```python
from build123d import *

# Parameters (mm, degrees)
F0_R      = 7.25
F1_DEPTH  = 14
F3_R      = 3
F4_DEPTH  = 14.001
F6_R      = 12.75
F7_DEPTH  = 25
F8_R      = 3.95
F9_DEPTH  = 39.001
F10_R     = 12.75
F10_R_2   = 11.5
F11_DEPTH = 20
F13_DEPTH = 5
F14_R     = 3.95
F15_DEPTH = 6.5


with BuildPart() as f1:
    # F0 (on Front) → F1 (new body)
    with BuildSketch(Plane.XZ):
        Circle(F0_R)
    extrude(amount=F1_DEPTH)

    # F3 (on face) → F4 (cut, through all)
    with BuildSketch(Plane.XZ.offset(14)):
        Circle(F3_R)
    extrude(amount=-F4_DEPTH, mode=Mode.SUBTRACT)

    # F6 (on offset) → F7 (join)
    with BuildSketch(Plane(origin=(0, 0, 0), x_dir=(-1, 0, 0), z_dir=(0, 1, 0))):
        Circle(F6_R)
    extrude(amount=F7_DEPTH)

    # F8 (on face) → F9 (cut, through all)
    with BuildSketch(Plane(origin=(0, 25, 0), x_dir=(-1, 0, 0), z_dir=(0, 1, 0))):
        Circle(F8_R)
    extrude(amount=-F9_DEPTH, mode=Mode.SUBTRACT)

    # F10 (on face) → F11 (cut)
    with BuildSketch(Plane(origin=(0, 25, 0), x_dir=(-1, 0, 0), z_dir=(0, 1, 0))):
        Circle(F10_R)
        Circle(F10_R_2, mode=Mode.SUBTRACT)
    extrude(amount=-F11_DEPTH, mode=Mode.SUBTRACT)

    # F12 (on face) → F13 (join)
    with BuildSketch(Plane(origin=(0, 5, 0), x_dir=(-1, 0, 0), z_dir=(0, 1, 0))):
        with BuildLine():
            ThreePointArc((2, 12.5921602595), (0, 12.75), (-2, 12.5921602595))
            Line((-2, 12.5921602595), (-2, 11.3247516529))
            ThreePointArc((-2, 11.3247516529), (0, 11.5), (2, 11.3247516529))
            Line((2, 11.3247516529), (2, 12.5921602595))
        make_face()
        with BuildLine():
            Line((-2, -11.3247516529), (-2, -12.5921602595))
            ThreePointArc((-2, -12.5921602595), (0, -12.75), (2, -12.5921602595))
            Line((2, -12.5921602595), (2, -11.3247516529))
            ThreePointArc((2, -11.3247516529), (0, -11.5), (-2, -11.3247516529))
        make_face()
    extrude(amount=F13_DEPTH)

    # F14 (on face) → F15 (cut)
    with BuildSketch(Plane(origin=(0, 25, 0), x_dir=(-1, 0, 0), z_dir=(0, 1, 0))):
        Polygon((5.6975970229, 5.0613622835), (-1.5344698039, 7.4649449041), (-7.2320668267, 2.4035826206), (-5.6975970229, -5.0613622835), (1.5344698039, -7.4649449041), (7.2320668267, -2.4035826206), align=None)
        Circle(F14_R, mode=Mode.SUBTRACT)
    extrude(amount=-F15_DEPTH, mode=Mode.SUBTRACT)


solid = f1.part
```
CAD build for the part. Positions are in the model's coordinates, mm. A direction names the side the tool comes from. Round coordinates to 2 decimals unless told otherwise and drop trailing zeros. Order: outer loops, then holes, each group sorted by start corner. A loop starts at its lowest first (then second) coordinate and runs counter-clockwise, first axis right, second up. Notation, with made-up numbers: (29, 45.5) - (82, 45.5) arc R30 ccw to (82, 75.5) - close; hole circle Ø5 at (40, 12). An arc over 180 degrees is marked (long way). Answer in a Markdown table with one row per item. Add a question column.
(1) 3-axis set-ups, long thin cutter, end or side, ignore diameter. For faces 1 (the face through (3.35, -6.9, -6.43)), 2 (the face through (-2, 7, -12)), 3 (the face through (2, 7, 12)), 4 (the face through (2, 7, -12)), 5 (the face through (6.476, 21.796, -1.277)): which of +Z, -Z, +X, -X, +Y, -Y reach the whole face in a straight line?
(2) Probe L1, parallel to Z at x = 0, y = -5.5; L2, parallel to Y at x = -1.25, z = -5; L3, parallel to Y at x = 10, z = -1. List the from-to ranges inside material, lowest first. Write a range as [from, to].
(3) Band-saw the part on B-B on y = 4.5. List the corners of the cut face in (x, z).
(4) Band-saw the part on C-C on z = 0. List the corners of the cut face in (x, y), and give its area (3 significant figures).
(5) Mould opens along Z. For faces 6 (the face through (-12, 5, 0)), 7 (the face through (3.135, 2.477, -2.404)), 8 (the face through (2.493, 15.14, -11.227)) say: +Z half, -Z half, draft (parallel to the pull), parting line (faces both ways), or undercut.
(6) Band-saw the part on D-D on x = -10.5. List the corners of the cut face in (y, z), and give its area (3 significant figures).
(7) Drop flat-ended pins along their axis: pin 1 Ø12 at (x, y) = (-10, -7.5) entering from +Z; pin 2 Ø1 at (y, z) = (8, 12) entering from +X; pin 3 Ø8 at (y, z) = (3.5, -4.5) entering from +X. Give the stop position or say it passes through.
(8) Band-saw the part on A-A on x = 0. List the corners of the cut face in (y, z), and give its area (3 significant figures).
Data:
| question | item | result |
|---|---|---|
| 1 | face 1 | -Y |
| 1 | face 2 | -Z, -X, +Y |
| 1 | face 3 | +Z, +X, +Y |
| 1 | face 4 | -Z, +X, +Y |
| 1 | face 5 | +Y |
| 2 | L1 | z = [-7.25, -3.95], [3.95, 7.25] |
| 2 | L2 | y = [-14, 18.5] |
| 2 | L3 | y = [0, 25] |
| 3 | outline | circle Ø25.5 at (0, 0); hole circle Ø7.9 at (0, 0) |
| 4 | outline | (-12.75, 0) - (-7.25, 0) - (-7.25, -14) - (-3.95, -14) - (-3.95, 18.5) - (-6.74, 18.5) - (-6.74, 25) - (-11.5, 25) - (-11.5, 5) - (-12.75, 5) - close; (3.95, -14) - (7.25, -14) - (7.25, 0) - (12.75, 0) - (12.75, 5) - (11.5, 5) - (11.5, 25) - (6.74, 25) - (6.74, 18.5) - (3.95, 18.5) - close |
| 4 | area | 446 mm^2 |
| 5 | face 6 | draft |
| 5 | face 7 | undercut |
| 5 | face 8 | parting line |
| 6 | outline | (0, -7.23) - (5, -7.23) - (5, -4.69) - (25, -4.69) - (25, 4.69) - (5, 4.69) - (5, 7.23) - (0, 7.23) - close |
| 6 | area | 260 mm^2 |
| 7 | pin 1 | stops at z = 6.05 |
| 7 | pin 2 | stops at x = 2 |
| 7 | pin 3 | stops at x = 12.74 |
| 8 | outline | (-14, -7.25) - (0, -7.25) - (0, -12.75) - (10, -12.75) - (10, -11.5) - (25, -11.5) - (25, -6.95) - (18.5, -6.95) - (18.5, -3.95) - (-14, -3.95) - close; (-14, 3.95) - (18.5, 3.95) - (18.5, 6.95) - (25, 6.95) - (25, 11.5) - (10, 11.5) - (10, 12.75) - (0, 12.75) - (0, 7.25) - (-14, 7.25) - close |
| 8 | area | 456 mm^2 |
